Autodesk Inventor part; units mm, degrees
ref_plane "YZ Plane" through (0, 0, 0) normal (1, 0, 0) x (0, 1, 0)
ref_plane "XZ Plane" through (0, 0, 0) normal (0, 1, 0) x (-1, 0, 0)
ref_plane "XY Plane" through (0, 0, 0) normal (0, 0, 1) x (1, 0, 0)
sketch "Sketch2" plane through (0, 0, 0) normal (0, 0, 1) x (1, 0, 0)
  line L0 (-10, -10) -> (-10, 110)
  line L1 (-10, 110) -> (10, 110)
  line L2 (10, 110) -> (50, 70)
  line L3 (50, 70) -> (50, -10)
  line L4 (50, -10) -> (-10, -10)
  circle A0 centre (40, 0) radius 2.5
  circle A1 centre (40, 20) radius 2.5
  circle A2 centre (40, 40) radius 2.5
  circle A3 centre (40, 60) radius 2.5
  circle A4 centre (20, 80) radius 2.5
  circle A5 centre (20, 60) radius 2.5
  circle A6 centre (20, 40) radius 2.5
  circle A7 centre (20, 20) radius 2.5
  circle A8 centre (20, 0) radius 2.5
  circle A9 centre (0, 0) radius 2.5
  circle A10 centre (0, 20) radius 2.5
  circle A11 centre (0, 40) radius 2.5
  circle A12 centre (0, 60) radius 2.5
  circle A13 centre (0, 80) radius 2.5
  circle A14 centre (0, 100) radius 2.5
extrude "Extrusion1" add sketch "Sketch2" along normal blind 5
properties part number "MAKERSLIDE_RISERS"
Part model, mm, in its own coordinate system. Give positions to 0.01 mm unless a question says otherwise; leave off trailing zeros. Loops run counter-clockwise (first coordinate to the right, second up) from the corner with the lowest first, then second, coordinate; pieces in that order, holes last. Notation, with made-up numbers: M -40,-7 L 17,-7 A24 ccw 17,27 Z; hole C -11.5,81 d6. An arc over 180 degrees is marked long. Put each result on its own line as item: value. Start each with the question number.
1) Probe probe 1 along Y at (x, z) = (40, 1.5); probe 2 along X at (y, z) = (40.5, 3.9); probe 3 along Y at (x, z) = (39, 0.35). List the from-to ranges inside material, lowest first.
2) Saw through at D-D (x = 0). List the corners of the cut face in (y, z).
3) Pull direction Y, two halves, no side cores. Call faces 1 (the cylindrical face through (-0.33, 97.52, 2.46)), 2 (the cylindrical face through (1.34, 57.89, 2.46)), 3 (the flat face through (50, 31, 2)), 4 (the flat face through (0, 110, 2)): +Y half, -Y half, draft (parallel to the pull), parting line (faces both ways), or undercut.
4) Saw through at B-B (x = 20). List the corners of the cut face in (y, z).
5) Saw through at C-C (y = 40). List the corners of the cut face in (x, z), then the cut area to 3 significant figures.
6) Saw through at A-A (y = 80). List the corners of the cut face in (x, z), then the cut area to 3 significant figures.
Numbers:
1. probe 1: -10 to -2.5, 2.5 to 17.5, 22.5 to 37.5, 42.5 to 57.5, 62.5 to 80
1. probe 2: -10 to -2.45, 2.45 to 17.55, 22.45 to 37.55, 42.45 to 50
1. probe 3: -10 to -2.29, 2.29 to 17.71, 22.29 to 37.71, 42.29 to 57.71, 62.29 to 81
2. outline: M -10,0 L -2.5,0 L -2.5,5 L -10,5 Z; M 2.5,0 L 17.5,0 L 17.5,5 L 2.5,5 Z; M 22.5,0 L 37.5,0 L 37.5,5 L 22.5,5 Z; M 42.5,0 L 57.5,0 L 57.5,5 L 42.5,5 Z; M 62.5,0 L 77.5,0 L 77.5,5 L 62.5,5 Z; M 82.5,0 L 97.5,0 L 97.5,5 L 82.5,5 Z; M 102.5,0 L 110,0 L 110,5 L 102.5,5 Z
3. face 1: undercut
3. face 2: undercut
3. face 3: draft
3. face 4: +Y half
4. outline: M -10,0 L -2.5,0 L -2.5,5 L -10,5 Z; M 2.5,0 L 17.5,0 L 17.5,5 L 2.5,5 Z; M 22.5,0 L 37.5,0 L 37.5,5 L 22.5,5 Z; M 42.5,0 L 57.5,0 L 57.5,5 L 42.5,5 Z; M 62.5,0 L 77.5,0 L 77.5,5 L 62.5,5 Z; M 82.5,0 L 100,0 L 100,5 L 82.5,5 Z
5. outline: M -10,0 L -2.5,0 L -2.5,5 L -10,5 Z; M 2.5,0 L 17.5,0 L 17.5,5 L 2.5,5 Z; M 22.5,0 L 37.5,0 L 37.5,5 L 22.5,5 Z; M 42.5,0 L 50,0 L 50,5 L 42.5,5 Z
5. area: 225 mm^2
6. outline: M -10,0 L -2.5,0 L -2.5,5 L -10,5 Z; M 2.5,0 L 17.5,0 L 17.5,5 L 2.5,5 Z; M 22.5,0 L 40,0 L 40,5 L 22.5,5 Z
6. area: 200 mm^2
